Check sheet for the modelled part. Datum: model origin and axes. Units: mm. A direction names the side the tool comes from. Round coordinates to 2 decimals unless told otherwise and drop trailing zeros. Loops run counter-clockwise (first coordinate to the right, second up) from the corner with the lowest first, then second, coordinate; pieces in that order, holes last. Notation, with made-up numbers: (-8.75, 79.5) -> (10.25, 79.5) arc R31 ccw to (10.25, 110.5) -> close; hole circle Ø8 at (-20, 12). An arc over 180 degrees is marked (long way). One line per item, written item: value. Start each with the question number.
1. Set-up check for faces 4 (the face through (2, -2, -16)), 5 (the face through (2, 8, -5)), 6 (the face through (10, 2.001, -16)): record each of +Z, -Z, +X, -X, +Y, -Y from which the full face is reachable in a straight line by a thin tool's end or side.
2. Go/stop test with flat-tipped pins: pin 1 (8 mm diameter, centred on x = 20.5, y = 4, fed in from -Z); pin 2 (3 mm diameter, centred on x = 1.5, z = -13, fed in from -Y); pin 3 (13 mm diameter, centred on x = 12.5, z = -8, fed in from +Y). Record where each tip stops, or that it passes through.
3. Cross-section at C-C on y = 5. Record the cut outline in (x, z).
4. Release check for a two-part mould opening along Y. For faces 1 (the face through (4, 14.2, -15.9)), 2 (the face through (22, 2, -16)), 3 (the face through (1.97, 8.84, -29.46)) record: +Y half, -Y half, draft (parallel to the pull), parting line (faces both ways), or undercut.
5. Cross-section at A-A on z = -16. Count the separate pieces of the cut face and the enclosed holes in it, then the cut area to 3 significant figures.
6. Cross-section at B-B on y = 8. Record the cut outline in (x, z).
7. Material ranges on L1, parallel to Z at x = 2, y = 10.5; L2, parallel to X at y = 0.5, z = -16; L3, parallel to Y at x = 2, z = -24, recorded low to high.
from build123d import *

# Parameters (mm, degrees)
SKETCH1_W                = 32
SKETCH1_H                = 16
SKETCH1_W_2              = 22
SKETCH1_H_2              = 12
BOSS_EXTRUDE1_DEPTH      = 4
SKETCH3_W                = 32
SKETCH3_H                = 2.001260946
BOSS_EXTRUDE3_DEPTH      = 12
BOSS_EXTRUDE5_DEPTH      = 4
BOSS_EXTRUDE5_DEPTH_BACK = 2
CHAMFER1_SIZE            = 4
SKETCH8_R                = 2.6
CUT_EXTRUDE2_DEPTH       = 50.477267507
SKETCH9_R                = 1
CUT_EXTRUDE3_DEPTH       = 49
CHAMFER2_SIZE            = 2


with BuildPart() as part:
    # Sketch1 → Boss-Extrude1 (new body)
    with BuildSketch(Plane(origin=(0, 0, 0), x_dir=(0, 0, -1), z_dir=(1, 0, 0))):
        with Locations((16, 8)):
            Rectangle(SKETCH1_W, SKETCH1_H)
        with Locations((16, 8)):
            Rectangle(SKETCH1_W_2, SKETCH1_H_2, mode=Mode.SUBTRACT)
    extrude(amount=BOSS_EXTRUDE1_DEPTH)

    # Sketch3 → Boss-Extrude3 (add)
    with BuildSketch(Plane(origin=(4, 0, 0), x_dir=(0, 0, -1), z_dir=(1, 0, 0))):
        with Locations((16, 1.000630473)):
            Rectangle(SKETCH3_W, SKETCH3_H)
    extrude(amount=BOSS_EXTRUDE3_DEPTH)

    # Sketch7 → Boss-Extrude5 (add, two sides: drawn at the far end of the back side and taken through both)
    with BuildSketch(Plane.XZ.offset(-BOSS_EXTRUDE5_DEPTH_BACK)):
        with BuildLine():
            Line((0, 0), (16, 0))
            ThreePointArc((16, 0), (32, -16), (16, -32))
            Line((16, -32), (0, -32))
            Line((0, -32), (0, 0))
        make_face()
    extrude(amount=BOSS_EXTRUDE5_DEPTH + BOSS_EXTRUDE5_DEPTH_BACK)

    # Chamfer1
    chamfer1_edges = [part.edges().sort_by_distance(p)[0] for p in [
        (0, -4, -16),
    ]]
    chamfer(chamfer1_edges, length=CHAMFER1_SIZE)

    # Sketch8 → Cut-Extrude2 (cut, through all)
    with BuildSketch(Plane.XZ.offset(4)):
        with Locations(Location((16, -16, 0), (0, 0, 270))):
            Circle(SKETCH8_R)
    extrude(amount=-CUT_EXTRUDE2_DEPTH, mode=Mode.SUBTRACT)

    # Sketch9 → Cut-Extrude3 (cut, through all)
    with BuildSketch(Plane.ZY):
        with Locations((-30, 8)):
            Circle(SKETCH9_R)
        with Locations((-2, 8)):
            Circle(SKETCH9_R)
    extrude(amount=-CUT_EXTRUDE3_DEPTH, mode=Mode.SUBTRACT)

    # Chamfer2
    chamfer2_edges = [part.edges().sort_by_distance(p)[0] for p in [
        (2, 16, 0),
        (2, 16, -32),
    ]]
    chamfer(chamfer2_edges, length=CHAMFER2_SIZE)


solid = part.part
Taken from the geometry:
1. face 4: +Z, -Z, -X, -Y
1. face 5: +X, -X
1. face 6: +Z, -Z, +X, +Y
2. pin 1: stops at z = -31.97
2. pin 2: stops at y = -3
2. pin 3: stops at y = 2
3. outline: (0, -32) -> (4, -32) -> (4, -27) -> (0, -27) -> close; (0, -5) -> (4, -5) -> (4, 0) -> (0, 0) -> close
4. face 1: draft
4. face 2: +Y half
4. face 3: undercut
5. separate pieces: 3
5. enclosed holes: 0
5. area: 161 mm2
6. outline: (0, -32) -> (4, -32) -> (4, -31) -> (0, -31) -> close; (0, -29) -> (4, -29) -> (4, -27) -> (0, -27) -> close; (0, -5) -> (4, -5) -> (4, -3) -> (0, -3) -> close; (0, -1) -> (4, -1) -> (4, 0) -> (0, 0) -> close
7. L1: z = -32 to -27, -5 to 0
7. L2: x = 0 to 13.4, 18.6 to 32
7. L3: y = -2 to 2, 14 to 16
